Source: CAD feature listing. Evaluate the final solid. Frame: model axes, mm. A direction names the side the tool comes from. Round coordinates to 2 decimals unless told otherwise and drop trailing zeros. Order: outer loops, then holes, each group sorted by start corner. A loop starts at its lowest first (then second) coordinate and runs counter-clockwise, first axis right, second up. Notation, with made-up numbers: (84, -35) - (132, -35) arc R20 cw to (132, -24) - close; hole circle Ø3 at (79, 84.5). An arc over 180 degrees is marked (long way). Return JSON: item names as keys, results as strings. Group by question number.
1) Contact query for flat-ended pins moving along their axis: P1, Ø3, axis at x = -3.5, y = -83.5, coming from the +Z side; P2, Ø5.5, axis at y = -78, z = -70, coming from the +X side; P3, Ø2, axis at y = -78.5, z = -58.5, coming from the -X side; P4, Ø1, axis at y = -85.5, z = -60.5, coming from the -X side. Output: stop coordinate, or through.
2) Section B-B, the plane y = -84.5. Return loops of the section in (x, z), plus the area to 3 significant figures.
3) Access query for faces 5 (the flat face through (0, -81, 0)), 6 (the flat face through (-15.958, -79, -74)), 7 (the flat face through (16.042, -79, -74)). Directions: +Z, -Z, +X, -X, +Y, -Y. A direction counts if a zero-diameter tool reaches every point of the face in a straight line with its end or side. Return the directions, or none.
4) Section A-A, the plane z = -41. Return loops of the section in (x, y).
5) Mould query, pull axis Y, two halves, no side actions, for faces 1 (the cylindrical face through (0.269, -94.486, -73.95)), 2 (the flat face through (0, -79, -150)), 3 (the conical face through (-0.125, -89.555, -73.95)), 4 (the flat face through (-16.65, -84.39, -76.05)). Classes: pulls with the +Y half, pulls with the -Y half, needs draft (parallel to the pull), parting line crosses it, or undercut.
6) Section C-C, the plane y = -78. Return loops of the section in (x, z).
7) Section D-D, the plane z = -68. Return loops of the section in (x, y), plus the area to 3 significant figures.
8) Ray query, line 1 (X direction, y = -86.25, z = -98); line 2 (Y direction, x = 4, z = -17); line 3 (Y direction, x = -6, z = -66). Return the intervals inside material, ascending. Write a range as from..to.
```python
from build123d import *

# Parameters (mm, degrees)
BOSS_EXTRUDE2_DEPTH = 150
CUT_EXTRUDE1_DEPTH  = 179.003087993
CUT_EXTRUDE1_DRAFT  = 0.75
BOSS_EXTRUDE3_DEPTH = 150


with BuildPart() as part:
    # Sketch1 → Boss-Extrude2 (new body)
    with BuildSketch(Plane.XY):
        with BuildLine():
            Line((-15.957671772, -92.173910335), (-15.957671772, -75.48673473))
            Line((-15.957671772, -75.48673473), (16.042328228, -75.48673473))
            Line((16.042328228, -75.48673473), (16.042328228, -92.173910335))
            ThreePointArc((16.042328228, -92.173910335), (0.042328228, -94.48673473), (-15.957671772, -92.173910335))
        make_face()
    extrude(amount=-BOSS_EXTRUDE2_DEPTH)


with BuildPart() as cut_extrude1_tool:
    # Sketch4 → Cut-Extrude1 (with draft: the straight prism first)
    with BuildSketch(Plane.XY):
        with BuildLine():
            Line((10.142328228, -87.568485405), (10.142328228, -81.38673473))
            Line((10.142328228, -81.38673473), (-10.057671772, -81.38673473))
            Line((-10.057671772, -81.38673473), (-10.057671772, -87.568485405))
            ThreePointArc((-10.057671772, -87.568485405), (0.042328228, -88.58673473), (10.142328228, -87.568485405))
        make_face()
    extrude(amount=-CUT_EXTRUDE1_DEPTH)
    # Cut-Extrude1: the draft: its side faces are tilted about the plane it starts from
    cut_extrude1_sides = [cut_extrude1_tool.faces().sort_by_distance(p)[0] for p in [
        (0.042328228, -88.58673473, -89.501543996),
        (10.142328228, -84.477610068, -89.501543996),
        (0.042328228, -81.38673473, -89.501543996),
        (-10.057671772, -84.477610068, -89.501543996),
    ]]
    draft(cut_extrude1_sides, Plane.XY, CUT_EXTRUDE1_DRAFT)


with BuildPart() as part_1:
    add(part.part)

    # Cut-Extrude1: cut by cut_extrude1_tool
    add(cut_extrude1_tool.part, mode=Mode.SUBTRACT)

    # Sketch5 → Boss-Extrude3 (add)
    with BuildSketch(Plane(origin=(0, 0, -150), x_dir=(-1, 0, 0), z_dir=(0, 0, -1))):
        with BuildLine():
            Line((-17.509626323, -90.700736876), (-16.042328228, -90.893910335))
            Line((-16.042328228, -90.893910335), (-16.042328228, -82.570693355))
            Line((-16.042328228, -82.570693355), (-17.447829646, -86.253845746))
            ThreePointArc((-17.447829646, -86.253845746), (-17.46006126, -86.306080257), (-17.457968161, -86.359686931))
            Line((-17.457968161, -86.359686931), (-17.126211232, -88.252050567))
            ThreePointArc((-17.126211232, -88.252050567), (-17.120591762, -88.338766729), (-17.133832096, -88.424650167))
            Line((-17.133832096, -88.424650167), (-17.67670625, -90.450684094))
            ThreePointArc((-17.67670625, -90.450684094), (-17.649815007, -90.61356195), (-17.509626323, -90.700736876))
        make_face()
        with BuildLine():
            Line((15.957671772, -90.893910335), (15.957671772, -82.570693355))
            Line((15.957671772, -82.570693355), (17.36317319, -86.253845746))
            ThreePointArc((17.36317319, -86.253845746), (17.375404804, -86.306080257), (17.373311704, -86.359686931))
            Line((17.373311704, -86.359686931), (17.041554775, -88.252050567))
            ThreePointArc((17.041554775, -88.252050567), (17.035935306, -88.338766729), (17.049175639, -88.424650167))
            Line((17.049175639, -88.424650167), (17.592049794, -90.450684094))
            ThreePointArc((17.592049794, -90.450684094), (17.565158551, -90.61356195), (17.424969867, -90.700736876))
            Line((17.424969867, -90.700736876), (15.957671772, -90.893910335))
        make_face()
    extrude(amount=-BOSS_EXTRUDE3_DEPTH)


solid = part_1.part
```
Geometry check:
{
 "1": {"P1": "through", "P2": "x = 16.04", "P3": "x = -15.96", "P4": "x = -17.27"},
 "2": {"outline": "(-16.69, -150) - (-12.02, -150) - (-10.06, 0) - (-16.69, 0) - close; (10.14, 0) - (12.11, -150) - (16.78, -150) - (16.78, 0) - close", "area": "1,700 mm2"},
 "3": {"face 5": "+Z, +X, -X, +Y, -Y", "face 6": "+Z, -Z, -X, +Y", "face 7": "+Z, -Z, +X, +Y"},
 "4": {"outline": "(-17.59, -90.45) arc R0.2 ccw to (-17.42, -90.7) - (-15.96, -90.89) - (-15.96, -92.17) arc R56.5 ccw to (16.04, -92.17) - (16.04, -90.89) - (17.51, -90.7) arc R0.2 ccw to (17.68, -90.45) - (17.13, -88.42) arc R0.4 cw to (17.13, -88.25) - (17.46, -86.36) arc R0.2 ccw to (17.45, -86.25) - (16.04, -82.57) - (16.04, -75.49) - (-15.96, -75.49) - (-15.96, -82.57) - (-17.36, -86.25) arc R0.2 ccw to (-17.37, -86.36) - (-17.04, -88.25) arc R0.4 cw to (-17.05, -88.42) - close; hole (-10.59, -88) arc R51.14 ccw to (10.68, -88) - (10.68, -80.85) - (-10.59, -80.85) - close"},
 "5": {"face 1": "pulls with the -Y half", "face 2": "needs draft", "face 3": "undercut", "face 4": "pulls with the +Y half"},
 "6": {"outline": "(-15.96, -150) - (16.04, -150) - (16.04, 0) - (-15.96, 0) - close"},
 "7": {"outline": "(-17.59, -90.45) arc R0.2 ccw to (-17.42, -90.7) - (-15.96, -90.89) - (-15.96, -92.17) arc R56.5 ccw to (16.04, -92.17) - (16.04, -90.89) - (17.51, -90.7) arc R0.2 ccw to (17.68, -90.45) - (17.13, -88.42) arc R0.4 cw to (17.13, -88.25) - (17.46, -86.36) arc R0.2 ccw to (17.45, -86.25) - (16.04, -82.57) - (16.04, -75.49) - (-15.96, -75.49) - (-15.96, -82.57) - (-17.36, -86.25) arc R0.2 ccw to (-17.37, -86.36) - (-17.04, -88.25) arc R0.4 cw to (-17.05, -88.42) - close; hole (-10.95, -88.29) arc R51.49 ccw to (11.03, -88.29) - (11.03, -80.5) - (-10.95, -80.5) - close", "area": "412 mm2"},
 "8": {"line 1": "-17.36..-11.34, 11.43..17.45", "line 2": "-94.35..-88.65, -81.16..-75.49", "line 3": "-94.16..-89.09, -80.52..-75.49"}
}
